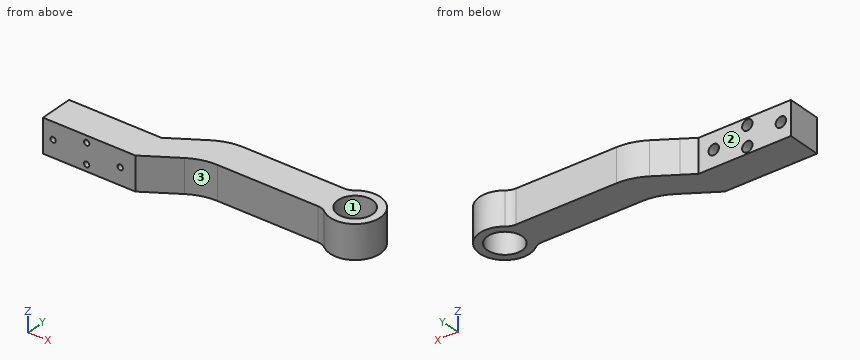
from build123d import *

# Parameters (mm, degrees)
MODEL_R             = 10.3
EXTRUDE_1_DEPTH     = 20
SKETCH_2_R          = 1.6
CUT_EXTRUDE_1_DEPTH = 22
SKETCH_4_R          = 3.1
CUT_EXTRUDE_2_DEPTH = 9
SKETCH_5_W          = 3
SKETCH_5_H          = 20
CUT_EXTRUDE_3_DEPTH = 22


with BuildPart() as part:
    # Model → 凸台-拉伸1 (new body)
    with BuildSketch(Plane.XY):
        with BuildLine():
            Line((233.591051214, 295.2839002), (226.237796851, 290.623912247))
            Line((226.237796851, 290.623912247), (217.532290693, 290.623912247))
            Line((217.532290693, 290.623912247), (168.237796851, 290.623912247))
            Line((168.237796851, 290.623912247), (168.237796851, 270.623912247))
            Line((168.237796851, 270.623912247), (226.237796851, 270.623912247))
            Line((226.237796851, 270.623912247), (245.869173527, 283.06493146))
            ThreePointArc((245.869173527, 283.06493146), (253.567322868, 286.536378604), (261.927934048, 287.724919413))
            Line((261.927934048, 287.724919413), (321.918709695, 287.724919413))
            ThreePointArc((321.918709695, 287.724919413), (324.556497218, 287.277539951), (326.899261749, 285.985438659))
            ThreePointArc((326.899261749, 285.985438659), (351.237796839, 297.723317855), (326.900192078, 309.463125896))
            ThreePointArc((326.900192078, 309.463125896), (324.557590785, 308.171303033), (321.920064905, 307.724039843))
            Line((321.920064905, 307.724039843), (261.928239839, 307.724854901))
            ThreePointArc((261.928239839, 307.724854901), (253.567416793, 306.536370888), (245.869071734, 303.06486695))
            Line((245.869071734, 303.06486695), (233.591051214, 295.2839002))
        make_face()
        with Locations((336.237796851, 297.723912247)):
            Circle(MODEL_R, mode=Mode.SUBTRACT)
    extrude(amount=EXTRUDE_1_DEPTH)

    # 草图2 → 切除-拉伸1 (cut)
    with BuildSketch(Plane(origin=(0, 270.623912247, 0), x_dir=(-1, 0, 0), z_dir=(0, -1, 0))):
        with Locations(Location((-177.237796851, -10, 0), (0, 0, 90))):
            Circle(SKETCH_2_R)
        with Locations(Location((-217.237796851, -10, 0), (0, 0, 90))):
            Circle(SKETCH_2_R)
        with Locations(Location((-197.237796851, -16, 0), (0, 0, 90))):
            Circle(SKETCH_2_R)
        with Locations(Location((-197.237796851, -4, 0), (0, 0, 90))):
            Circle(SKETCH_2_R)
    extrude(amount=-CUT_EXTRUDE_1_DEPTH, mode=Mode.SUBTRACT)

    # 草图4 → 切除-拉伸2 (cut)
    with BuildSketch(Plane(origin=(0, 290.623912247, 0), x_dir=(1, 0, 0), z_dir=(0, 1, 0))):
        with Locations(Location((177.237796851, -10, 0), (0, 0, 270))):
            Circle(SKETCH_4_R)
        with Locations(Location((197.237796851, -16, 0), (0, 0, 270))):
            Circle(SKETCH_4_R)
        with Locations(Location((197.237796851, -4, 0), (0, 0, 270))):
            Circle(SKETCH_4_R)
        with Locations(Location((217.237796851, -10, 0), (0, 0, 270))):
            Circle(SKETCH_4_R)
    extrude(amount=-CUT_EXTRUDE_2_DEPTH, mode=Mode.SUBTRACT)

    # 草图5 → 切除-拉伸3 (cut)
    with BuildSketch(Plane(origin=(0, 290.623912247, 0), x_dir=(1, 0, 0), z_dir=(0, 1, 0))):
        with Locations((169.737796851, -10)):
            Rectangle(SKETCH_5_W, SKETCH_5_H)
    extrude(amount=-CUT_EXTRUDE_3_DEPTH, mode=Mode.SUBTRACT)


solid = part.part
Design review of the part built by this model. Coordinates are the model's own, in mm. Face numbers are marked on the shaded views. A direction names the side the tool comes from. Coordinates: 2 decimals unless noted, no trailing zeros. Loops run counter-clockwise (first coordinate to the right, second up) from the corner with the lowest first, then second, coordinate; pieces in that order, holes last. Notation, with made-up numbers: M 40.25,54.25 L 86.25,54.25 A20 cw 86.25,59.25 Z; hole C 8,33.5 d7. An arc over 180 degrees is marked long. Use one line per item in the form item = value.
(1) Clearance check with flat-ended pins moving along their axes: P1, Ø3.5, axis at x = 177.24, z = 10, coming from the -Y side; P2, Ø10, axis at x = 293, z = 13.5, coming from the +Y side; P3, Ø5, axis at x = 217.5, z = 9.5, coming from the +Y side; P4, Ø2.5, axis at x = 177.24, z = 10, coming from the -Y side. State where each tip first meets the part, or that it passes through.
Return value:
P1 = 270.62
P2 = 307.72
P3 = 281.62
P4 = through
(2) Consider section C-C (y = 277). Write out the cut boundary in (x, z), and give its area (3 significant figures).
Return value:
outline = M 171.24,0 L 236.3,0 L 236.3,20 L 171.24,20 Z; hole C 177.24,10 d3.2; hole C 197.24,4 d3.2; hole C 197.24,16 d3.2; hole C 217.24,10 d3.2
area = 1,270 mm2
(3) Consider section D-D (x = 265). Write out the cut boundary in (y, z).
Return value:
outline = M 287.72,0 L 307.72,0 L 307.72,20 L 287.72,20 Z
(4) Consider section A-A (z = 10). Give the number of separate pieces and of enclosed holes in the cut face, and give its area (3 significant figures).
Return value:
separate_pieces = 3
enclosed_holes = 1
area = 3,220 mm2
(5) For line 1 along X through (y, z) = (288.5, 8.5); line 2 along X through (y, z) = (284.5, 16); line 3 along X through (y, z) = (285.5, 10), list the stretches that pass through material, from the lowest coordinate up. Write a range as from..to.
Return value:
line_1 = 171.24..174.52, 179.95..214.52, 219.95..331.65, 340.82..348.07
line_2 = 171.24..194.14, 200.34..248.4, 329.16..343.32
line_3 = 171.24..174.14, 180.34..214.14, 220.34..250.59, 327.54..344.93
(6) For the marked faces 1, 2 and 3, list the 3-axis set-ups (+Z, -Z, +X, -X, +Y, -Y) from which the entire face can be reached by the end or side of a thin tool; tool diameter is ignored.
Return value:
face_1 = +Z, -Z
face_2 = +Z, -Z, -X, +Y
face_3 = +Z, -Z, -Y
(7) Consider section B-B (y = 301). Write out the cut boundary in (x, z).
Return value:
outline = M 242.61,0 L 326.47,0 L 326.47,20 L 242.61,20 Z; M 346,0 L 350.88,0 L 350.88,20 L 346,20 Z
